```python
from build123d import *

# Parameters (mm, degrees)
BOSS_EXTRUDE1_DEPTH     = 44
FILLET1_R               = 6
SKETCH2_R               = 2.05
CUT_EXTRUDE1_DEPTH      = 46.782092569
LPATTERN1_COUNT         = 3
LPATTERN1_PITCH         = 8
MIRROR1_COPY_1_SKETCH_R = 2.05
MIRROR1_COPY_1_DEPTH    = 46.782092569
MIRROR1_COPY_2_SKETCH_R = 2.05
MIRROR1_COPY_2_DEPTH    = 46.782092569


with BuildPart() as part:
    # Sketch1 → Boss-Extrude1 (new body)
    with BuildSketch(Plane.XY):
        Polygon((0, 0), (4, 0), (4, 2), (3, 2), (3, 10), (4, 10), (4, 12), (0, 12), align=None)
    extrude(amount=-BOSS_EXTRUDE1_DEPTH)

    # Fillet1
    fillet1_edges = [part.edges().sort_by_distance(p)[0] for p in [
        (2, 12, 0),
        (2, 0, 0),
        (2, 0, -44),
        (2, 12, -44),
    ]]
    fillet(fillet1_edges, radius=FILLET1_R - 0.0001)  # a hair under: the kernel refuses the full size

    # Sketch2 → Cut-Extrude1 (cut, through all)
    with BuildSketch(Plane.ZY):
        with Locations(Location((-38, 6, 0), (0, 0, 270))):
            Circle(SKETCH2_R)
    cut_extrude1 = extrude(amount=-CUT_EXTRUDE1_DEPTH, mode=Mode.SUBTRACT)

    # LPattern1: Cut-Extrude1 ×3
    with Locations(*[(0, 0, i * LPATTERN1_PITCH) for i in range(1, LPATTERN1_COUNT)]):
        add(cut_extrude1, mode=Mode.SUBTRACT)

    # Mirror1: Cut-Extrude1 across plane
    add(cut_extrude1.mirror(Plane.XY.offset(-22)), mode=Mode.SUBTRACT)

    # Mirror1 copy 1 sketch → Mirror1 copy 1 (cut, through all)
    with BuildSketch(Plane(origin=(0, 0, -52), x_dir=(0, 0, -1), z_dir=(-1, 0, 0))):
        with Locations((-38, -6)):
            Circle(MIRROR1_COPY_1_SKETCH_R)
    extrude(amount=-MIRROR1_COPY_1_DEPTH, mode=Mode.SUBTRACT)

    # Mirror1 copy 2 sketch → Mirror1 copy 2 (cut, through all)
    with BuildSketch(Plane(origin=(0, 0, -60), x_dir=(0, 0, -1), z_dir=(-1, 0, 0))):
        with Locations((-38, -6)):
            Circle(MIRROR1_COPY_2_SKETCH_R)
    extrude(amount=-MIRROR1_COPY_2_DEPTH, mode=Mode.SUBTRACT)


solid = part.part
```
Here's how the part is built. I have some questions about the finished solid (model axes, mm). A direction names the side the tool comes from. Coordinates: 2 decimals unless noted, no trailing zeros. Order: outer loops, then holes, each group sorted by start corner. A loop starts at its lowest first (then second) coordinate and runs counter-clockwise, first axis right, second up.
1) We'd pull the mould along Y, two halves only. Please class faces 1 (the face through (1.972, 10.289, -42.196)), 2 (the face through (1.479, 6.267, -27.967)), 3 (the face through (2.028, 1.711, -1.804)): +Y half, -Y half, draft (parallel to the pull), parting line (faces both ways), or undercut.
2) Imagine slicing it at D-D on z = -19.5. List the corners of the cut face in (x, y) for me, and give its area (3 significant figures).
3) Will these pins go through, and if not, where does the flat tip stop? pin 1 (4 mm diameter, centred on y = 5, z = -22.5, fed in from +X); pin 2 (1.5 mm diameter, centred on x = 1, y = 8, fed in from -Z); pin 3 (1 mm diameter, centred on x = 1.5, y = 7, fed in from +Z).
4) Imagine slicing it at C-C on y = 4.75. List the corners of the cut face in (x, z) for me, and give its area (3 significant figures).
5) Imagine slicing it at B-B on x = 1.1. State how many separate pieces and enclosed holes the cut face has, and give its area (3 significant figures).
6) Which directions (+Z, -Z, +X, -X, +Y, -Y) give clear straight access to the entire face, cutting with the end or side of a thin tool? Please do faces 4 (the face through (3.5, 10, -21.7)), 5 (the face through (1.48, 5.91, -11.95)).
7) Imagine slicing it at A-A on z = -30. List the corners of the cut face in (x, y) for me.
8) I need wall thicknesses on line 1 (Z direction, x = 1, y = 6); line 2 (Y direction, x = 1.65, z = -6); line 3 (Y direction, x = 3.75, z = -9.5). Which ranges of each line are inside material? Lowest first, please.
Response values:
1. face 1: +Y half
1. face 2: undercut
1. face 3: -Y half
2. outline: (0, 0) - (4, 0) - (4, 2) - (3, 2) - (3, 10) - (4, 10) - (4, 12) - (0, 12) - close
2. area: 40.0 mm2
3. pin 1: stops at x = 3
3. pin 2: stops at z = -43.87
3. pin 3: stops at z = -0.02
4. outline: (0, -43.87) - (3, -43.87) - (3, -39.62) - (0, -39.62) - close; (0, -36.38) - (3, -36.38) - (3, -31.62) - (0, -31.62) - close; (0, -28.38) - (3, -28.38) - (3, -23.62) - (0, -23.62) - close; (0, -20.38) - (3, -20.38) - (3, -15.62) - (0, -15.62) - close; (0, -12.38) - (3, -12.38) - (3, -7.62) - (0, -7.62) - close; (0, -4.38) - (3, -4.38) - (3, -0.13) - (0, -0.13) - close
4. area: 82.5 mm2
5. separate pieces: 1
5. enclosed holes: 5
5. area: 431 mm2
6. face 4: +Z, -Z, +X
6. face 5: +X, -X
7. outline: (0, 0) - (4, 0) - (4, 2) - (3, 2) - (3, 3.95) - (0, 3.95) - close; (0, 8.05) - (3, 8.05) - (3, 10) - (4, 10) - (4, 12) - (0, 12) - close
8. line 1: z = -44 to -40.05, -35.95 to -32.05, -27.95 to -24.05, -19.95 to -16.05, -11.95 to -8.05, -3.95 to 0
8. line 2: y = 0 to 3.95, 8.05 to 12
8. line 3: y = 0 to 2, 10 to 12
